Drawing for the job (mm, zero at the part's lowest x, y, z). A direction names the side the tool comes from. Coordinates: 2 decimals unless noted, no trailing zeros. Order: outer loops, then holes, each group sorted by start corner. A loop starts at its lowest first (then second) coordinate and runs counter-clockwise, first axis right, second up.
1) Cut at C-C (x = 63). List the corners of the cut face in (y, z) (3 decimals).
2) Cut at A-A (y = 6.35). List the corners of the cut face in (x, z) (3 decimals), and give its area (3 significant figures).
3) Wall check: L1, parallel to X at y = 6.35, z = 23.3; L2, parallel to Y at x = 15.5, z = 8.5 (3 decimals). Give the ranges that are in metal, low to high.
4) Mould opens along Y. For the marked faces 3, 4 and 5 say: +Y half, -Y half, draft (parallel to the pull), parting line (faces both ways), or undercut.
5) Cut at B-B (z = 5.5). List the corners of the cut face in (x, y) (3 decimals).
6) Cut at D-D (y = 38.1). List the corners of the cut face in (x, z) (1 decimal).
7) Tool access for the marked faces 1 and 2: list every direction of +Z, -Z, +X, -X, +Y, -Y with a clear straight run to the whole face (end or side of a thin tool).
8) Pin check, flat tips, straight feed: pin 1 Ø6 at (x, y) = (6.35, 69.85) entering from -Z; pin 2 Ø3 at (x, y) = (69.85, 69.85) entering from +Z. Stop position of each tip, or through.
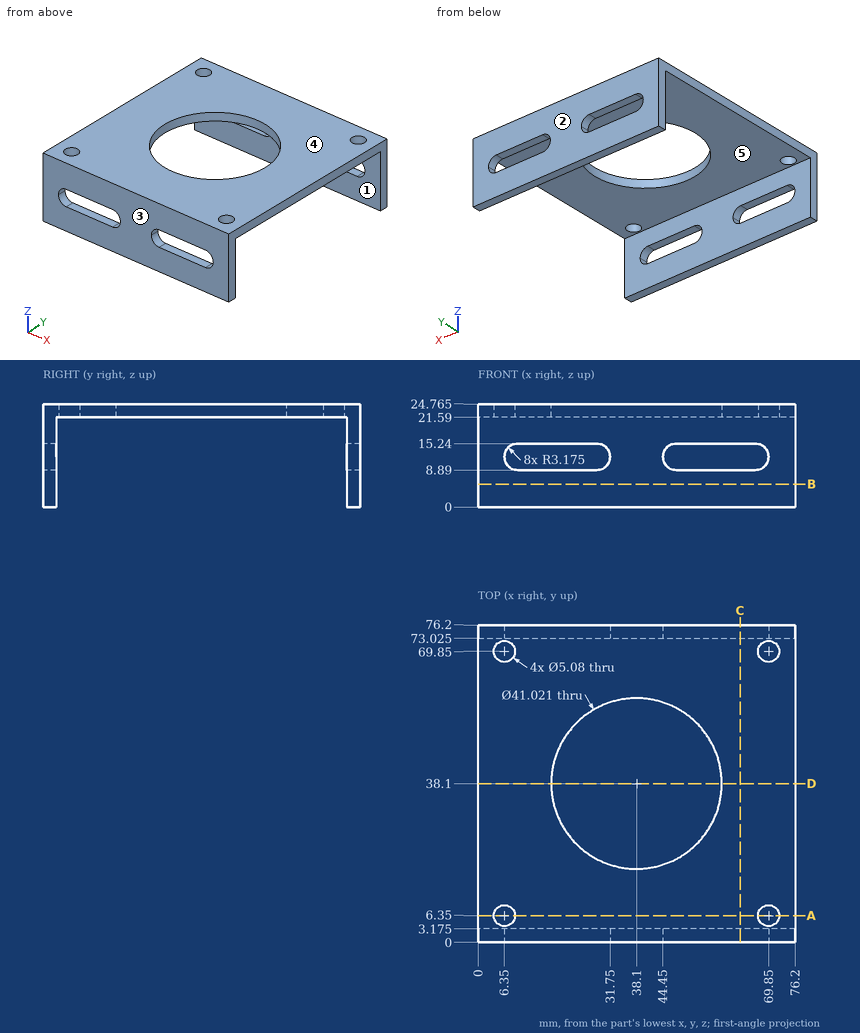
Geometry check:
1. outline: (0, 0) - (3.175, 0) - (3.175, 8.89) - (0, 8.89) - close; (0, 15.24) - (3.175, 15.24) - (3.175, 21.59) - (73.025, 21.59) - (73.025, 15.24) - (76.2, 15.24) - (76.2, 24.765) - (0, 24.765) - close; (73.025, 0) - (76.2, 0) - (76.2, 8.89) - (73.025, 8.89) - close
2. outline: (0, 21.59) - (3.81, 21.59) - (3.81, 24.765) - (0, 24.765) - close; (8.89, 21.59) - (67.31, 21.59) - (67.31, 24.765) - (8.89, 24.765) - close; (72.39, 21.59) - (76.2, 21.59) - (76.2, 24.765) - (72.39, 24.765) - close
2. area: 210 mm2
3. L1: x = 0 to 3.81, 8.89 to 67.31, 72.39 to 76.2
3. L2: y = 0 to 3.175, 73.025 to 76.2
4. face 3: -Y half
4. face 4: draft
4. face 5: undercut
5. outline: (0, 0) - (76.2, 0) - (76.2, 3.175) - (0, 3.175) - close; (0, 73.025) - (76.2, 73.025) - (76.2, 76.2) - (0, 76.2) - close
6. outline: (0, 21.6) - (17.6, 21.6) - (17.6, 24.8) - (0, 24.8) - close; (58.6, 21.6) - (76.2, 21.6) - (76.2, 24.8) - (58.6, 24.8) - close
7. face 1: -Z, +X, -X
7. face 2: +Z, -Z, +X, -X, +Y
8. pin 1: stops at z = 21.59
8. pin 2: passes through
